Build history of the part. All positions in model axes, mm. Coordinates: 2 decimals unless noted, no trailing zeros. Write each loop counter-clockwise with the first axis right and the second up, starting at its lowest first coordinate (ties: lowest second). Pieces come first, ordered by that corner, then holes.
```python
from build123d import *

# Parameters (mm, degrees)
F0_R     = 28.7655
F0_R_2   = 36.195
F1_DEPTH = 5.08
F3_D     = 6.7564
F5_D     = 3.175
F7_D     = 3.175
F9_D     = 9.525


with BuildPart() as f1:
    # F0 (on Top) → F1 (new body)
    with BuildSketch(Plane.XY):
        with BuildLine():
            Line((152.4, 0), (12.7, 0))
            ThreePointArc((12.7, 0), (3.7197438789, -3.7197438789), (0, -12.7))
            Line((0, -12.7), (0, -177.8))
            ThreePointArc((0, -177.8), (3.7197438789, -186.7802561211), (12.7, -190.5))
            Line((12.7, -190.5), (152.4, -190.5))
            ThreePointArc((152.4, -190.5), (161.3802561211, -186.7802561211), (165.1, -177.8))
            Line((165.1, -177.8), (165.1, -12.7))
            ThreePointArc((165.1, -12.7), (161.3802561211, -3.7197438789), (152.4, 0))
        make_face()
        with Locations((82.55, -133.35)):
            Circle(F0_R, mode=Mode.SUBTRACT)
        with Locations((82.55, -47.625)):
            Circle(F0_R_2, mode=Mode.SUBTRACT)
    extrude(amount=F1_DEPTH)

    # F3 (through all)
    with Locations(Plane.XY.offset(5.08)):
        with Locations((8.2098719395, -8.2098719395), (156.8901280605, -8.2098719395), (156.8901280605, -182.2901280605), (8.2098719395, -182.2901280605)):
            Hole(F3_D / 2)

    # F5 (through all)
    with Locations(Plane.XY.offset(5.08)):
        with Locations((14.2875, -185.7248), (150.8125, -185.7248), (150.8125, -4.7752), (14.2875, -4.7752)):
            Hole(F5_D / 2)

    # F7 (through all)
    with Locations(Plane.XY.offset(5.08)):
        with Locations((29.21, -82.55), (29.21, -12.7), (135.89, -12.7), (135.89, -82.55)):
            Hole(F7_D / 2)

    # F9 (through all)
    with Locations(Plane.XY.offset(5.08)):
        with Locations((22.479, -47.625)):
            Hole(F9_D / 2)


solid = f1.part
```
1. Saw through at C-C on z = 0.9. State how many separate pieces and enclosed holes the cut face has, plus the area to 3 significant figures.
Computed values:
separate pieces: 1
enclosed holes: 15
area: 24,300 mm2
2. Saw through at D-D on y = -138.5. List the corners of the cut face in (x, z).
Computed values:
outline: (0, 0) - (54.25, 0) - (54.25, 5.08) - (0, 5.08) - close; (110.85, 0) - (165.1, 0) - (165.1, 5.08) - (110.85, 5.08) - close
3. Probe line 1 along Y through (x, z) = (135.89, 3.5); line 2 along Y through (x, z) = (97.5, 3.8); line 3 along Y through (x, z) = (24, 1.8). List the from-to ranges inside material, lowest first.
Computed values:
line 1: y = -190.5 to -84.14, -80.96 to -14.29, -11.11 to 0
line 2: y = -190.5 to -157.93, -108.77 to -80.59, -14.66 to 0
line 3: y = -190.5 to -52.14, -43.11 to 0
4. Saw through at A-A on x = 82.55. List the corners of the cut face in (y, z).
Computed values:
outline: (-190.5, 0) - (-162.12, 0) - (-162.12, 5.08) - (-190.5, 5.08) - close; (-104.58, 0) - (-83.82, 0) - (-83.82, 5.08) - (-104.58, 5.08) - close; (-11.43, 0) - (0, 0) - (0, 5.08) - (-11.43, 5.08) - close
5. Saw through at B-B on y = -75.5. List the corners of the cut face in (x, z), plus the area to 3 significant figures.
Computed values:
outline: (0, 0) - (59.46, 0) - (59.46, 5.08) - (0, 5.08) - close; (105.64, 0) - (165.1, 0) - (165.1, 5.08) - (105.64, 5.08) - close
area: 604 mm2
6. Mould opens along Y. For faces 1 (the face through (117.074, -36.753, 2.504)), 2 (the face through (3.62, -186.68, 2.5)), 3 (the face through (165.1, -96, 3)) say: +Y half, -Y half, draft (parallel to the pull), parting line (faces both ways), or undercut.
Computed values:
face 1: undercut
face 2: -Y half
face 3: draft
